Verification items for this drawing (mm, ordinates from the low corner). A direction names the side the tool comes from. Coordinates: 2 decimals unless noted, no trailing zeros. Write each loop counter-clockwise with the first axis right and the second up, starting at its lowest first coordinate (ties: lowest second). Pieces come first, ordered by that corner, then holes. Notation, with made-up numbers: M 63,-33.75 L 119,-33.75 A30 cw 119,5.25 Z; hole C 70,-31 d4. An arc over 180 degrees is marked long. Write each question's results on one line, items separated by ' | '.
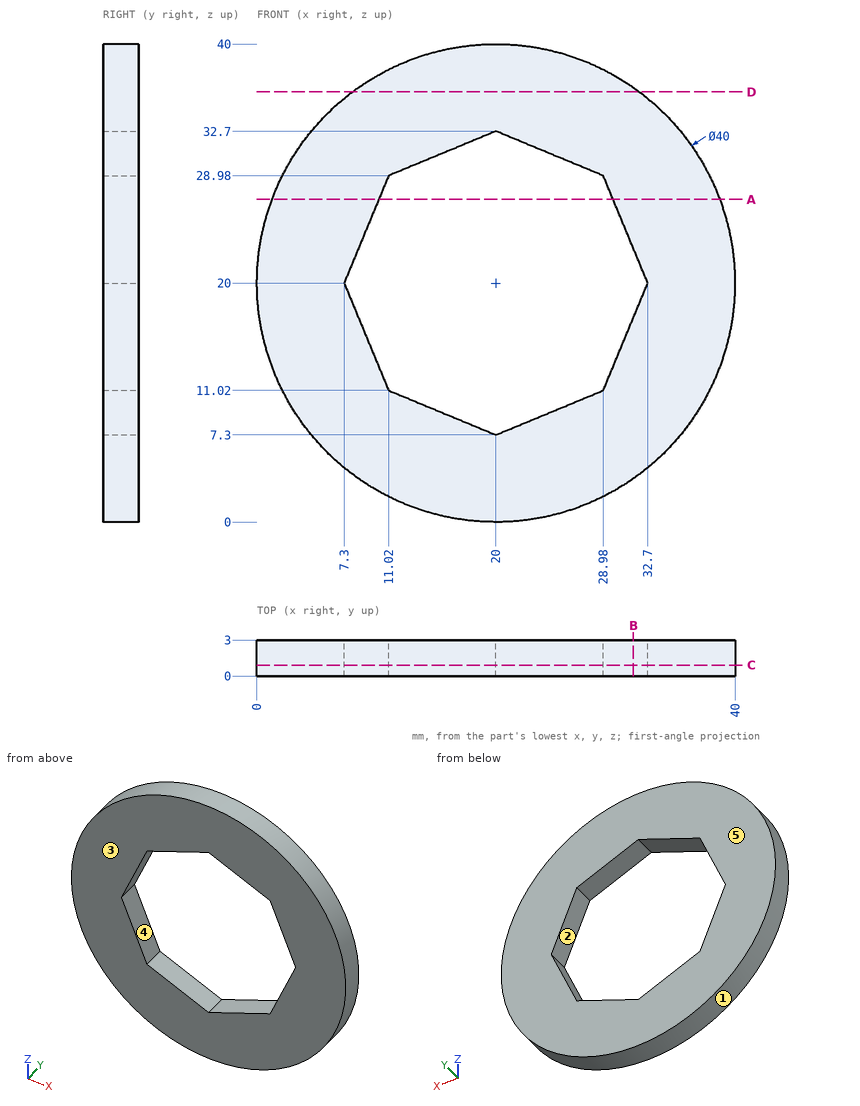
Q1. Scan lines: probe 1 along Z at (x, y) = (20, 2.5); probe 2 along X at (y, z) = (1.5, 29) (1 decimal); probe 3 along X at (y, z) = (2.05, 19.5). Record each from-to range of solid material in increasing order.
Geometry check:
probe 1: z = 0 to 7.3, 32.7 to 40 | probe 2: x = 2.1 to 11.1, 28.9 to 37.9 | probe 3: x = 0.01 to 7.51, 32.49 to 39.99
Q2. Sectioned sample at A-A on z = 27. Record the cut outline in (x, y) (1 decimal), and give its area (3 significant figures).
Geometry check:
outline: M 1.3,0 L 10.2,0 L 10.2,3 L 1.3,3 Z; M 29.8,0 L 38.7,0 L 38.7,3 L 29.8,3 Z | area: 53.6 mm2
Q3. Mould release check, pull along X, two halves, no side actions. Record for the marked faces 1, 2 and 3: pulls with the +X half, pulls with the -X half, needs draft (parallel to the pull), parting line crosses it, or undercut.
Geometry check:
face 1: parting line crosses it | face 2: undercut | face 3: needs draft
Q4. Depth check by flat-ended pin: P1, Ø12, axis at x = 23, z = 24, coming from the -Y side. Enter the tip coordinate at first touch or a pass-through.
Geometry check:
P1: passes through
Q5. Sectioned sample at C-C on y = 0.9. Record the cut outline in (x, z).
Geometry check:
outline: C 20,20 d40; hole M 7.3,20 L 11.02,11.02 L 20,7.3 L 28.98,11.02 L 32.7,20 L 28.98,28.98 L 20,32.7 L 11.02,28.98 Z
Q6. Sectioned sample at B-B on x = 31.5. Record the cut outline in (y, z).
Geometry check:
outline: M 0,3.64 L 3,3.64 L 3,17.1 L 0,17.1 Z; M 0,22.9 L 3,22.9 L 3,36.36 L 0,36.36 Z
Q7. Access from +Z, -Z, +X, -X, +Y, -Y to the whole of each face (thin tool, end or side, straight path). Record for the marked faces 4 and 5.
Geometry check:
face 4: +Y, -Y | face 5: +Z, -Z, +X, -X, +Y
Q8. Sectioned sample at D-D on z = 36. Record the cut outline in (x, y), and give its area (3 significant figures).
Geometry check:
outline: M 8,0 L 32,0 L 32,3 L 8,3 Z | area: 72.0 mm2
